```python
from build123d import *

# Parameters (mm, degrees)
F0_W          = 15.8
F0_H          = 15.8
F1_DEPTH      = 9.5
F0_R          = 3.05
F2_DEPTH      = 1
F0_R_2        = 2.25
F3_DEPTH      = 1.9
F3_DEPTH_BACK = 0.1
F4_DEPTH      = 8.9


with BuildPart() as f1:
    # F0 (on Top) → F1 (new body)
    with BuildSketch(Plane.XY):
        Rectangle(F0_W, F0_H)
        Polygon((3.95, 6.4), (6.4, 6.4), (6.4, 3.95), (6.4, -3.95), (6.4, -6.4), (3.95, -6.4), (-3.95, -6.4), (-6.4, -6.4), (-6.4, -3.95), (-6.4, 3.95), (-6.4, 6.4), (-3.95, 6.4), align=None, mode=Mode.SUBTRACT)
    extrude(amount=-F1_DEPTH)

    # F0 (on Top) → F2 (join)
    with BuildSketch(Plane.XY):
        with BuildLine():
            ThreePointArc((6.4, 3.95), (2.2175883861, 2.2175883861), (3.95, 6.4))
            Line((3.95, 6.4), (-3.95, 6.4))
            ThreePointArc((-3.95, 6.4), (-2.2175883861, 5.6824116139), (-1.5, 3.95))
            ThreePointArc((-1.5, 3.95), (-3.95, 1.5), (-6.4, 3.95))
            Line((-6.4, 3.95), (-6.4, -3.95))
            ThreePointArc((-6.4, -3.95), (-3.95, -1.5), (-1.5, -3.95))
            ThreePointArc((-1.5, -3.95), (-2.2175883861, -5.6824116139), (-3.95, -6.4))
            Line((-3.95, -6.4), (3.95, -6.4))
            ThreePointArc((3.95, -6.4), (2.2175883861, -2.2175883861), (6.4, -3.95))
            Line((6.4, -3.95), (6.4, 3.95))
        make_face()
        Circle(F0_R, mode=Mode.SUBTRACT)
        with BuildLine():
            ThreePointArc((-6.4, 3.95), (-5.6824116139, 5.6824116139), (-3.95, 6.4))
            Line((-3.95, 6.4), (-6.4, 6.4))
            Line((-6.4, 6.4), (-6.4, 3.95))
        make_face()
        with BuildLine():
            Line((6.4, 3.95), (6.4, 6.4))
            Line((6.4, 6.4), (3.95, 6.4))
            ThreePointArc((3.95, 6.4), (5.6824116139, 5.6824116139), (6.4, 3.95))
        make_face()
        with BuildLine():
            Line((6.4, -6.4), (6.4, -3.95))
            ThreePointArc((6.4, -3.95), (5.6824116139, -5.6824116139), (3.95, -6.4))
            Line((3.95, -6.4), (6.4, -6.4))
        make_face()
        with BuildLine():
            ThreePointArc((-3.95, -6.4), (-5.6824116139, -5.6824116139), (-6.4, -3.95))
            Line((-6.4, -3.95), (-6.4, -6.4))
            Line((-6.4, -6.4), (-3.95, -6.4))
        make_face()
    extrude(amount=-F2_DEPTH)

    # F0 (on Top) → F3 (join, two sides)
    with BuildSketch(Plane.XY) as f3_sk:
        with BuildLine():
            ThreePointArc((-1.5, -3.95), (-3.95, -1.5), (-6.4, -3.95))
            ThreePointArc((-6.4, -3.95), (-5.6824116139, -5.6824116139), (-3.95, -6.4))
            ThreePointArc((-3.95, -6.4), (-2.2175883861, -5.6824116139), (-1.5, -3.95))
        make_face()
        with BuildLine():
            ThreePointArc((-1.5, 3.95), (-2.2175883861, 5.6824116139), (-3.95, 6.4))
            ThreePointArc((-3.95, 6.4), (-5.6824116139, 5.6824116139), (-6.4, 3.95))
            ThreePointArc((-6.4, 3.95), (-3.95, 1.5), (-1.5, 3.95))
        make_face()
        with BuildLine():
            ThreePointArc((6.4, 3.95), (5.6824116139, 5.6824116139), (3.95, 6.4))
            ThreePointArc((3.95, 6.4), (2.2175883861, 2.2175883861), (6.4, 3.95))
        make_face()
        with BuildLine():
            ThreePointArc((3.95, -6.4), (5.6824116139, -5.6824116139), (6.4, -3.95))
            ThreePointArc((6.4, -3.95), (2.2175883861, -2.2175883861), (3.95, -6.4))
        make_face()
    extrude(amount=F3_DEPTH)
    extrude(f3_sk.sketch, amount=-F3_DEPTH_BACK)



with BuildPart() as f2:
    # F0 (on Top) → F2, piece 2 (new body)
    with BuildSketch(Plane.XY):
        Circle(F0_R_2)
    extrude(amount=-F2_DEPTH)


with BuildPart() as f1_1:
    add(f1.part)

    add(f2.part)  # F4 merges F2
    # F0 (on Top) → F4 (join)
    with BuildSketch(Plane.XY):
        Circle(F0_R)
        Circle(F0_R_2, mode=Mode.SUBTRACT)
    extrude(amount=-F4_DEPTH)


solid = f1_1.part
```
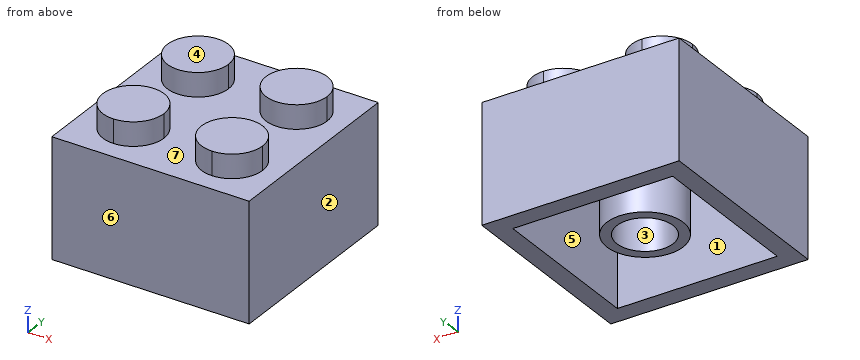
Geometry check sheet. Reference: the model listing, model coordinates, mm. Face numbers are marked on the shaded views. A direction names the side the tool comes from. Coordinates: 2 decimals unless noted, no trailing zeros. Loops run counter-clockwise (first coordinate to the right, second up) from the corner with the lowest first, then second, coordinate; pieces in that order, holes last.
Item 1: Go/stop test with flat-tipped pins: pin 1 Ø1 at (x, y) = (5, 0) entering from -Z; pin 2 Ø5.5 at (x, y) = (-4, -4) entering from -Z; pin 3 Ø1.2 at (x, y) = (-4.5, -5.5) entering from -Z; pin 4 Ø6.5 at (x, y) = (-1, 1.5) entering from -Z. Record where each tip stops, or that it passes through.
Item 2: Sectioned sample at A-A, the plane z = -1.75. Record the boundary of the cut face in (x, y), then the cut area to 3 significant figures.
Item 3: Sectioned sample at B-B, the plane z = -0.5. Record the boundary of the cut face in (x, y).
Item 4: Access from +Z, -Z, +X, -X, +Y, -Y to the whole of each face (thin tool, end or side, straight path). Record for the marked faces 5, 6 and 7.
Item 5: Thickness scan on line 1 (X direction, y = -3.95, z = -0.7); line 2 (Y direction, x = 0, z = -4.5). Record the ranges inside material, lowest first.
Item 6: Sectioned sample at C-C, the plane y = 0. Record the boundary of the cut face in (x, z), then the cut area to 3 significant figures.
Item 7: Release check for a two-part mould opening along X. For the marked faces 1, 2, 3 and 4 record: released by +X, released by -X, zero draft, split by the parting line, or undercut.
Check result:
1. pin 1: stops at z = -1
1. pin 2: stops at z = -9.5
1. pin 3: stops at z = -0.1
1. pin 4: stops at z = -8.9
2. outline: (-7.9, -7.9) - (7.9, -7.9) - (7.9, 7.9) - (-7.9, 7.9) - close; circle Ø6.1 at (0, 0); hole (-6.4, -6.4) - (6.4, -6.4) - (6.4, 6.4) - (-6.4, 6.4) - close; hole circle Ø4.5 at (0, 0)
2. area: 99.1 mm2
3. outline: (-7.9, -7.9) - (7.9, -7.9) - (7.9, 7.9) - (-7.9, 7.9) - close; hole circle Ø4.9 at (-3.95, -3.95); hole circle Ø4.9 at (-3.95, 3.95); hole circle Ø4.9 at (3.95, -3.95); hole circle Ø4.9 at (3.95, 3.95)
4. face 5: -Z
4. face 6: +Z, -Z, +X, -X, -Y
4. face 7: +Z
5. line 1: x = -7.9 to -6.4, -1.5 to 1.5, 6.4 to 7.9
5. line 2: y = -7.9 to -6.4, -3.05 to -2.25, 2.25 to 3.05, 6.4 to 7.9
6. outline: (-7.9, -9.5) - (-6.4, -9.5) - (-6.4, -1) - (-3.05, -1) - (-3.05, -8.9) - (-2.25, -8.9) - (-2.25, -1) - (2.25, -1) - (2.25, -8.9) - (3.05, -8.9) - (3.05, -1) - (6.4, -1) - (6.4, -9.5) - (7.9, -9.5) - (7.9, 0) - (-7.9, 0) - close
6. area: 53.9 mm2
7. face 1: undercut
7. face 2: released by +X
7. face 3: undercut
7. face 4: zero draft
